Geometry check sheet. Reference: the model listing, model coordinates, mm. Face numbers are marked on the shaded views. A direction names the side the tool comes from. Round coordinates to 2 decimals unless told otherwise and drop trailing zeros. Order: outer loops, then holes, each group sorted by start corner. A loop starts at its lowest first (then second) coordinate and runs counter-clockwise, first axis right, second up. Notation, with made-up numbers: (39.25, 10) - (88.25, 10) arc R9 ccw to (88.25, 26) - close; hole circle Ø3 at (3, 12). An arc over 180 degrees is marked (long way). Write each question's results on one line, items separated by ' | '.
```python
from build123d import *

# Parameters (mm, degrees)
EXTRUDE_1_DEPTH      = 12
CUT_EXTRUDE_12_DEPTH = 1
CUT_EXTRUDE_13_DEPTH = 1
CUT_EXTRUDE_14_DEPTH = 2.5
CUT_EXTRUDE_16_DEPTH = 2.5
SKETCH_26_R          = 1.5
CUT_EXTRUDE_17_DEPTH = 54.695511127
SKETCH_27_R          = 2
CUT_EXTRUDE_18_DEPTH = 54.151469748


with BuildPart() as part:
    # 스케치1 → 보스-돌출1 (new body)
    with BuildSketch(Plane.XY):
        Polygon((-11.994395335, 44.774969809), (-11.994395335, -5.625030191), (-13.999795062, -5.625030191), (-13.999795062, -26.825030191), (-9.199795062, -26.825030191), (-9.199795062, -8.525030191), (9.300204823, -8.527085749), (9.300204823, -26.827085749), (14.100204823, -26.827085749), (14.100204823, -5.627085749), (12.005604665, -5.627085749), (12.005604665, 44.774969809), align=None)
    extrude(amount=EXTRUDE_1_DEPTH)

    # 스케치20 → 컷-돌출12 (cut)
    with BuildSketch(Plane(origin=(14.100204823, 0, 0), x_dir=(0, 0, -1), z_dir=(1, 0, 0))):
        Polygon((-4.384999641, -23.626174282), (-7.614999641, -23.626174282), (-9.228415158, -20.82434965), (-7.61341897, -18.03073805), (-4.380259285, -18.03073805), (-2.768420518, -20.829824529), align=None)
    extrude(amount=-CUT_EXTRUDE_12_DEPTH, mode=Mode.SUBTRACT)

    # 스케치21 → 컷-돌출13 (cut)
    with BuildSketch(Plane.ZY.offset(13.999795062)):
        Polygon((7.611839128, -23.624116045), (4.381839128, -23.624116045), (2.768423611, -20.822291413), (4.383419799, -18.028679813), (7.616579484, -18.028679813), (9.228418251, -20.827766292), align=None)
    extrude(amount=-CUT_EXTRUDE_13_DEPTH, mode=Mode.SUBTRACT)

    # 스케치22 → 컷-돌출14 (cut)
    with BuildSketch(Plane.ZY.offset(-9.300204823)):
        Polygon((7.615000359, -23.624118724), (4.385000359, -23.624118724), (2.771584842, -20.822294093), (4.38658103, -18.028682492), (7.619740715, -18.028682492), (9.231579482, -20.827768971), align=None)
    extrude(amount=-CUT_EXTRUDE_14_DEPTH, mode=Mode.SUBTRACT)

    # 스케치25 → 컷-돌출16 (cut)
    with BuildSketch(Plane(origin=(-9.199795062, 0, 0), x_dir=(0, 0, -1), z_dir=(1, 0, 0))):
        Polygon((-4.384999641, -23.626174282), (-7.614999641, -23.626174282), (-9.228415158, -20.82434965), (-7.61341897, -18.03073805), (-4.380259285, -18.03073805), (-2.768420518, -20.829824529), align=None)
    extrude(amount=-CUT_EXTRUDE_16_DEPTH, mode=Mode.SUBTRACT)

    # 스케치26 → 컷-돌출17 (cut, through all)
    with BuildSketch(Plane.ZY.offset(12.999795062)):
        with Locations((6, -20.825030191)):
            Circle(SKETCH_26_R)
    extrude(amount=-CUT_EXTRUDE_17_DEPTH, mode=Mode.SUBTRACT)

    # 스케치27 → 컷-돌출18 (cut, through all)
    with BuildSketch(Plane(origin=(12.005604665, 0, 0), x_dir=(0, 0, -1), z_dir=(1, 0, 0))):
        with Locations(Location((-3, 38.972914251, 0), (0, 0, 90))):
            Circle(SKETCH_27_R)
    extrude(amount=-CUT_EXTRUDE_18_DEPTH, mode=Mode.SUBTRACT)


solid = part.part
```
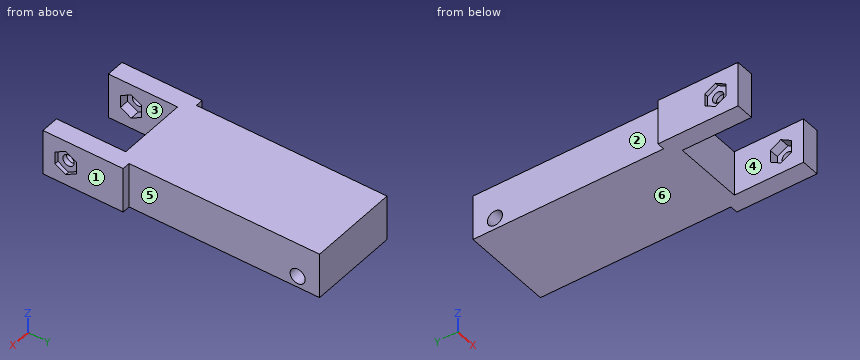
(1) Section check A-A (z = 11.25). Record the cut outline in (x, y).
Answers follow:
outline: (-14, -26.83) - (-9.2, -26.83) - (-9.2, -8.53) - (9.3, -8.53) - (9.3, -26.83) - (14.1, -26.83) - (14.1, -5.63) - (12.01, -5.63) - (12.01, 44.77) - (-11.99, 44.77) - (-11.99, -5.63) - (-14, -5.63) - close
(2) Draft check along X on the marked faces 3, 4, 5 and 6. Enter one of: released by +X, released by -X, zero draft, split by the parting line, or undercut.
Answers follow:
face 3: undercut | face 4: undercut | face 5: released by +X | face 6: zero draft
(3) Section check B-B (x = -11). Record the cut outline in (y, z) (3 decimals), then the cut area to 3 significant figures.
Answers follow:
outline: (-26.825, 0) - (44.775, 0) - (44.775, 12) - (-26.825, 12) - close; hole (-23.626, 4.385) - (-20.83, 2.768) - (-18.031, 4.38) - (-18.031, 7.613) - (-20.824, 9.228) - (-23.626, 7.615) - close; hole circle Ø4 at (38.973, 3) | area: 820 mm²
(4) Material ranges on line 1 (Y direction, x = -11.95, z = 6); line 2 (Y direction, x = 12.75, z = 6); line 3 (X direction, y = -22, z = 7.25), recorded low to high.
Answers follow:
line 1: -26.83 to -22.33, -19.33 to 44.77 | line 2: -26.83 to -22.33, -19.33 to -5.63 | line 3: -13 to -11.7, 11.8 to 13.1
(5) Section check D-D (y = 15). Record the cut outline in (x, z).
Answers follow:
outline: (-11.99, 0) - (12.01, 0) - (12.01, 12) - (-11.99, 12) - close
(6) Depth check by flat-ended pin: pin 1 Ø1 at (x, z) = (-13.5, 8.5) entering from +Y; pin 2 Ø6 at (y, z) = (33, 5.5) entering from +X; pin 3 Ø3.5 at (y, z) = (13, 7.5) entering from -X. Enter the tip coordinate at first touch or a pass-through.
Answers follow:
pin 1: y = -5.63 | pin 2: x = 12.01 | pin 3: x = -11.99
(7) Section check C-C (x = 5.75). Record the cut outline in (y, z).
Answers follow:
outline: (-8.53, 0) - (44.77, 0) - (44.77, 12) - (-8.53, 12) - close; hole circle Ø4 at (38.97, 3)
(8) Access from +Z, -Z, +X, -X, +Y, -Y to the whole of each face (thin tool, end or side, straight path). Record for the marked faces 1 and 2.
Answers follow:
face 1: +Z, -Z, +X, +Y, -Y | face 2: +Z, -Z, -X, +Y
